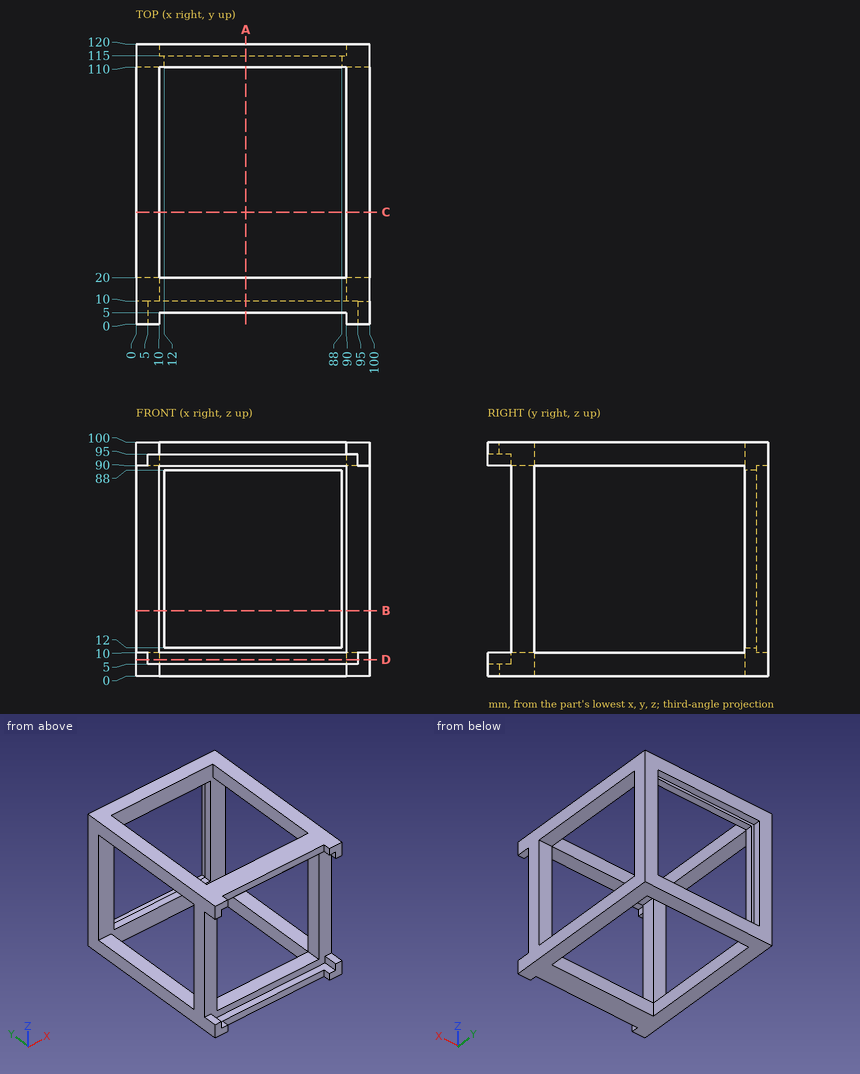
Geometry check sheet. Reference: drawing and pictorial views, mm from the part's lowest x, y, z. Round coordinates to 2 decimals unless told otherwise and drop trailing zeros. Write each loop counter-clockwise with the first axis right and the second up, starting at its lowest first coordinate (ties: lowest second). Pieces come first, ordered by that corner, then holes.
(1) Material ranges on line 1 (Z direction, x = 70, y = 17); line 2 (Y direction, x = 83.5, z = 7.5); line 3 (Z direction, x = 78, y = 110.5), recorded low to high.
Returned:
line 1: z = 0 to 10, 90 to 100
line 2: y = 10 to 20, 110 to 120
line 3: z = 0 to 12, 88 to 100
(2) Section check B-B (z = 28). Enter the section's corners in (x, y), plus the area to 3 significant figures.
Returned:
outline: (0, 10) - (10, 10) - (10, 20) - (0, 20) - close; (0, 110) - (12, 110) - (12, 115) - (10, 115) - (10, 120) - (0, 120) - close; (88, 110) - (100, 110) - (100, 120) - (90, 120) - (90, 115) - (88, 115) - close; (90, 10) - (100, 10) - (100, 20) - (90, 20) - close
area: 420 mm2
(3) Depth check by flat-ended pin: pin 1 Ø2.5 at (x, z) = (62.5, 1.5) entering from -Y. Enter the tip coordinate at first touch or a pass-through.
Returned:
pin 1: stops at y = 5
(4) Section check D-D (z = 7). Enter the section's corners in (x, y).
Returned:
outline: (0, 0) - (5, 0) - (5, 10) - (95, 10) - (95, 0) - (100, 0) - (100, 120) - (0, 120) - close; hole (10, 20) - (90, 20) - (90, 110) - (10, 110) - close
(5) Section check C-C (y = 48). Enter the section's corners in (x, z).
Returned:
outline: (0, 0) - (10, 0) - (10, 10) - (0, 10) - close; (0, 90) - (10, 90) - (10, 100) - (0, 100) - close; (90, 0) - (100, 0) - (100, 10) - (90, 10) - close; (90, 90) - (100, 90) - (100, 100) - (90, 100) - close
(6) Section check A-A (x = 47). Enter the section's corners in (y, z).
Returned:
outline: (5, 0) - (20, 0) - (20, 10) - (10, 10) - (10, 5) - (5, 5) - close; (5, 95) - (10, 95) - (10, 90) - (20, 90) - (20, 100) - (5, 100) - close; (110, 0) - (120, 0) - (120, 10) - (115, 10) - (115, 12) - (110, 12) - close; (110, 88) - (115, 88) - (115, 90) - (120, 90) - (120, 100) - (110, 100) - close
